Part model, mm, in its own coordinate system. A direction names the side the tool comes from. Round coordinates to 2 decimals unless told otherwise and drop trailing zeros. Loops run counter-clockwise (first coordinate to the right, second up) from the corner with the lowest first, then second, coordinate; pieces in that order, holes last. Notation, with made-up numbers: (-29, 50.5) -> (19, 50.5) arc R17 ccw to (19, 71.5) -> close; hole circle Ø1 at (89.25, 80.25). An arc over 180 degrees is marked (long way). Answer as a JSON object with one key per item and string values. Group by question number.
from build123d import *

# Parameters (mm, degrees)
F1_DEPTH = 2.5
F2_R     = 2.7521630024
F3_DEPTH = 1.5
F4_R     = 1.5
F5_DEPTH = 4


# Not quite as in the source:
# - a fillet or chamfer that OpenCascade refuses, or shapes differently, is made with other operations: its cross-section is extruded or revolved along the edge and cut away or added


with BuildPart() as f1:
    # F0 (on Front) → F1 (new body)
    with BuildSketch(Plane.XZ):
        Polygon((0, -3.1779241005), (2.7521630024, -1.5889620503), (2.7521630024, 1.5889620503), (0, 3.1779241005), (-2.7521630024, 1.5889620503), (-2.7521630024, -1.5889620503), align=None)
    extrude(amount=F1_DEPTH)

    # F2 (on face) → F3 (join)
    with BuildSketch(Plane.XZ.offset(2.5)):
        Circle(F2_R)
    extrude(amount=F3_DEPTH)

    # F4 (on face) → F5 (cut, through all)
    with BuildSketch(Plane.XZ.offset(4)):
        Circle(F4_R)
    extrude(amount=-F5_DEPTH, mode=Mode.SUBTRACT)

    # F6: fillet of radius 1.5 on 1 edges, made by hand

    # F6_s1 → F6_t2 (revolve, cut)
    with BuildSketch(Plane.XY):
        with BuildLine():
            ThreePointArc((2.7521630024, -2.5206160665), (2.3970986985, -3.4896992682), (1.5, -4))
            Line((1.5, -4), (2.7521630024, -4))
            Line((2.7521630024, -4), (2.7521630024, -2.5206160665))
        make_face()
    revolve(axis=Axis((0, -4, 0), (0, -1, 0)), mode=Mode.SUBTRACT)


solid = f1.part
Item 1: Which spindle directions (+Z, -Z, +X, -X, +Y, -Y) get a long thin tool onto all of the face, cutting with end or side? Do faces 1 (the face through (2.5, -2.5, 1.5)), 2 (the face through (-2.5, -2.5, 1.5)), 3 (the face through (-2.5, -2.5, -1.5)), 4 (the face through (2.5, -2.5, -1.5)). Say none if no direction does.
Item 2: Band-saw the part on A-A, the plane y = -1. List the corners of the cut face in (x, z).
Item 3: Drill centre lines: line 1 (X direction, y = -3.5, z = -0.25); line 2 (Z direction, x = 1.1, y = -3.7); line 3 (X direction, y = -1.8, z = 0.25). Where is each one in solid material? Low to high.
Item 4: Two-plate mould, pull along Z, no slides. Class faces 5 (the face through (-1.5, -2.03, 0.07)), 6 (the face through (2.752, -1, 0)), 7 (the face through (1.4, -1.23, 2.37)): pulls with the +Z half, pulls with the -Z half, needs draft (parallel to the pull), parting line crosses it, or undercut.
Item 5: Band-saw the part on B-B, the plane z = -3. List the corners of the cut face in (x, y).
Item 6: Drop flat-ended pins along their axis: pin 1 Ø1.1 at (x, z) = (-2, -1) entering from -Y; pin 2 Ø1.1 at (x, z) = (2.5, 1) entering from -Y; pin 3 Ø2 at (x, y) = (-2, -0.5) entering from -Z. Give the stop position or say it passes through.
Entries:
{
 "1": {"face 1": "+Z, +X, -Y", "face 2": "+Z, -X, -Y", "face 3": "-Z, -X, -Y", "face 4": "-Z, +X, -Y"},
 "2": {"outline": "(-2.75, -1.59) -> (0, -3.18) -> (2.75, -1.59) -> (2.75, 1.59) -> (0, 3.18) -> (-2.75, 1.59) -> close; hole circle Ø3 at (0, 0)"},
 "3": {"line 1": "-2.38 to -1.48, 1.48 to 2.38", "line 2": "-1.88 to -1.02, 1.02 to 1.88", "line 3": "-2.75 to -1.48, 1.48 to 2.75"},
 "4": {"face 5": "undercut", "face 6": "needs draft", "face 7": "pulls with the +Z half"},
 "5": {"outline": "(-0.31, -2.5) -> (0.31, -2.5) -> (0.31, 0) -> (-0.31, 0) -> close"},
 "6": {"pin 1": "y = -3.96", "pin 2": "y = -3.73", "pin 3": "z = -2.6"}
}
